from build123d import *

# Parameters (mm, degrees)
SKETCH1_5_W         = 15
SKETCH1_5_H         = 2.5
BOSS_EXTRUDE3_DEPTH = 2.5


with BuildPart() as part:
    # Sketch1_5 → Boss-Extrude3 (new body)
    with BuildSketch(Plane(origin=(0, 0, 0), x_dir=(0, 0, -1), z_dir=(1, 0, 0))):
        Polygon((-32.5, -25.5), (-25, -25.5), (-10, -25.5), (10, -25.5), (25, -25.5), (32.5, -25.5), (32.5, -20), (35, -20), (35, -10), (32.5, -10), (32.5, 10), (35, 10), (35, 20), (32.5, 20), (32.5, 25), (-32.5, 25), (-32.5, 20), (-35, 20), (-35, 10), (-32.5, 10), (-32.5, -10), (-35, -10), (-35, -20), (-32.5, -20), align=None)
        with Locations((-17.5, -26.75)):
            Rectangle(SKETCH1_5_W, SKETCH1_5_H)
        with Locations((17.5, -26.75)):
            Rectangle(SKETCH1_5_W, SKETCH1_5_H)
    extrude(amount=BOSS_EXTRUDE3_DEPTH)


solid = part.part
Input: part model. Units: mm. Frame: model coordinates. A direction names the side the tool comes from. Coordinates: 2 decimals unless noted, no trailing zeros. Order: outer loops, then holes, each group sorted by start corner. A loop starts at its lowest first (then second) coordinate and runs counter-clockwise, first axis right, second up. Notation, with made-up numbers: M 10.5,21 L 48.5,21 A14 ccw 48.5,35 Z; hole C 6.25,38.5 d2. An arc over 180 degrees is marked long. One line per question, with ' | ' between items.
Item 1: Section A-A (x = 1.05). Output: boundary loops of the cut face in (y, z).
Geometry results:
outline: M -28,-25 L -25.5,-25 L -25.5,-32.5 L -20,-32.5 L -20,-35 L -10,-35 L -10,-32.5 L 10,-32.5 L 10,-35 L 20,-35 L 20,-32.5 L 25,-32.5 L 25,32.5 L 20,32.5 L 20,35 L 10,35 L 10,32.5 L -10,32.5 L -10,35 L -20,35 L -20,32.5 L -25.5,32.5 L -25.5,25 L -28,25 L -28,10 L -25.5,10 L -25.5,-10 L -28,-10 Z
Item 2: Reachability of faces 1 (the flat face through (1, -10, -34)), 2 (the flat face through (1, -23, 32.5)), 3 (the flat face through (1, -25.5, 0)) from +Z, -Z, +X, -X, +Y, -Y: full face, straight path, thin tool, end or side. Return the list, or none.
Geometry results:
face 1: -Z, +X, -X | face 2: +Z, +X, -X, -Y | face 3: +X, -X, -Y
Item 3: Section C-C (y = -9). Output: boundary loops of the cut face in (x, z).
Geometry results:
outline: M 0,-32.5 L 2.5,-32.5 L 2.5,32.5 L 0,32.5 Z
Item 4: Pin query (flat end, axial travel): pin 1 (1.2 mm diameter, centred on x = 1, z = 30, fed in from -Y); pin 2 (0.8 mm diameter, centred on x = 1.5, z = -33.5, fed in from -Y); pin 3 (1.2 mm diameter, centred on x = 1.5, z = -34, fed in from +Y). Return the tip coordinate at first contact, or that it passes through.
Geometry results:
pin 1: stops at y = -25.5 | pin 2: stops at y = -20 | pin 3: stops at y = 20
Item 5: Ray query, line 1 along Z through (x, y) = (1.2, -2); line 2 along Y through (x, z) = (1.85, 3.5). Return the intervals inside material, ascending.
Geometry results:
line 1: z = -32.5 to 32.5 | line 2: y = -25.5 to 25
Item 6: Section B-B (z = 26.5). Output: boundary loops of the cut face in (x, y).
Geometry results:
outline: M 0,-25.5 L 2.5,-25.5 L 2.5,25 L 0,25 Z
Item 7: Draft query along Y for faces 4 (the flat face through (1, -10, 34)), 5 (the flat face through (1, 15, -35)), 6 (the flat face through (1, -20, -34)). Return one class per face: released by +Y, released by -Y, zero draft, split by the parting line, or undercut.
Geometry results:
face 4: undercut | face 5: zero draft | face 6: released by -Y
